Check sheet for the modelled part. Datum: model origin and axes. Units: mm. A direction names the side the tool comes from. Coordinates: 2 decimals unless noted, no trailing zeros. Write each loop counter-clockwise with the first axis right and the second up, starting at its lowest first coordinate (ties: lowest second). Pieces come first, ordered by that corner, then holes. Notation, with made-up numbers: (56, 32.25) -> (90, 32.25) arc R16 ccw to (90, 50.25) -> close; hole circle Ø3 at (31.5, 87.5). An arc over 180 degrees is marked (long way). One line per item, written item: value. Start each with the question number.
1) Scan lines: line 1 along Y through (x, z) = (12, 6); line 2 along X through (y, z) = (10, 3); line 3 along Y through (x, z) = (17, 9). Record each from-to range of solid material in increasing order. Write a range as [from, to].
2) Sectioned sample at A-A on z = 6. Enter the section's corners in (x, y).
3) Draft check along Y on faces 1 (the flat face through (-15, 15, 40)), 2 (the flat face through (-15, 8, 82)), 3 (the flat face through (10, 8, 6)). Enter one of: +Y half, -Y half, draft (parallel to the pull), parting line (faces both ways), or undercut.
4) Set-up check for faces 4 (the cylindrical face through (15.07, 3.595, 6.867)), 5 (the flat face through (-15, 0, 40)): record each of +Z, -Z, +X, -X, +Y, -Y from which the full face is reachable in a straight line by a thin tool's end or side.
5) Sectioned sample at B-B on x = 12. Enter the section's corners in (y, z), plus the area to 3 significant figures.
Autodesk Inventor part; units mm, degrees
ref_plane "YZ Plane" through (0, 0, 0) normal (1, 0, 0) x (0, 1, 0)
ref_plane "XZ Plane" through (0, 0, 0) normal (0, 1, 0) x (-1, 0, 0)
ref_plane "XY Plane" through (0, 0, 0) normal (0, 0, 1) x (1, 0, 0)
sketch "Sketch1" plane through (0, 0, 0) normal (0, 0, 1) x (1, 0, 0)
  line L0 (0, 0) -> (20, 0)
  line L1 (20, 0) -> (20, 15)
  line L2 (20, 15) -> (0, 15)
  line L3 (0, 15) -> (0, 0)
  dimension "d0" = 20
  dimension "d1" = 15
extrude "Extrusion1" add sketch "Sketch1" along normal blind 12
sketch "Sketch2" plane through (20, 0, 0) normal (1, 0, 0) x (0, 0, -1)
  circle A0 centre (-6, 7.5) radius 4
  point P0 (0, 0)
  dimension "d4" = 8
extrude "Extrusion2" cut sketch "Sketch2" against normal blind 10
sketch "Sketch3" plane through (0, 0, 12) normal (0, 0, 1) x (1, 0, 0)
  line L0 (4.6713, 10.3664) -> (9.2786, 10.3664)
  line L1 (9.2786, 10.3664) -> (9.2786, 7.6788)
  line L2 (9.2786, 7.6788) -> (4.6713, 7.6788)
  line L3 (4.6713, 7.6788) -> (4.6713, 10.3664)
  point P0 (0, 0)
extrude "Extrusion3" add sketch "Sketch3" along normal blind 10
sketch "Sketch4" plane through (0, 0, 12) normal (0, 0, 1) x (1, 0, 0)
  line L0 (20, 0) -> (20, 15)
  line L1 (0, 15) -> (0, 0)
  line L2 (20, 15) -> (0, 15)
  line L3 (0, 15) -> (0, 0)
  line L4 (0, 0) -> (20, 0)
  line L5 (20, 0) -> (20, 15)
extrude "Extrusion4" add sketch "Sketch4" along normal blind 50
sketch "Sketch5" plane through (0, 0, 0) normal (-1, 0, 0) x (0, 0, 1)
  line L0 (0, 15) -> (62, 15)
  line L1 (0, 0) -> (62, 0)
  line L2 (62, 0) -> (62, 15)
  line L3 (62, 15) -> (0, 15)
  line L4 (0, 15) -> (0, 0)
extrude "Extrusion5" add sketch "Sketch5" along normal blind 50
sketch "Sketch6" plane through (0, 0, 62) normal (0, 0, 1) x (1, 0, 0)
  line L0 (20, 0) -> (20, 15)
  line L1 (20, 15) -> (-50, 15)
  line L2 (20, 0) -> (-50, 0)
  line L3 (-50, 0) -> (-50, 15)
  line L4 (-50, 15) -> (20, 15)
  line L5 (20, 15) -> (20, 0)
  point P0 (0, 0)
extrude "Extrusion6" add sketch "Sketch6" along normal blind 20
properties part number "closing"
Answers:
1. line 1: y = [0, 3.5], [11.5, 15]
1. line 2: x = [-50, 10]
1. line 3: y = [0, 4.85], [10.15, 15]
2. outline: (-50, 0) -> (20, 0) -> (20, 3.5) -> (10, 3.5) -> (10, 11.5) -> (20, 11.5) -> (20, 15) -> (-50, 15) -> close
3. face 1: +Y half
3. face 2: draft
3. face 3: undercut
4. face 4: +X
4. face 5: +Z, -Z, +X, -X, -Y
5. outline: (0, 0) -> (15, 0) -> (15, 82) -> (0, 82) -> close; hole circle Ø8 at (7.5, 6)
5. area: 1,180 mm2
